```python
from build123d import *

# Parameters (mm, degrees)
SKETCH_1_W           = 32
SKETCH_1_H           = 11
EXTRUDE_1_DEPTH      = 1.6
SKETCH_2_W           = 0.64
SKETCH_2_H           = 0.64
EXTRUDE_2_DEPTH      = 6
SKETCH_3_W           = 0.64
SKETCH_3_H           = 0.64
EXTRUDE_3_DEPTH      = 8
FILLET_2_R           = 1
FILLET_3_R           = 1
FILLET_4_R           = 1
FILLET_5_R           = 1
SKETCH_4_W           = 8
SKETCH_4_H           = 11
EXTRUDE_4_DEPTH      = 8.4
FILLET_START         = 9
FILLET_4_2_OUTLINE_W = 6
FILLET_4_2_OUTLINE_H = 13
FILLET_4_2_DEPTH     = 1.960155108
FILLET_START_2       = 28.637824638
FILLET_5_2_OUTLINE_W = 5
FILLET_5_2_OUTLINE_H = 13
FILLET_5_2_DEPTH     = 2.362175362
SKETCH_5_R           = 1.25
CUT_EXTRUDE_1_DEPTH  = 6
SKETCH_6_W           = 2.5
SKETCH_6_H           = 2.5
EXTRUDE_5_DEPTH      = 2
SKETCH_7_W           = 0.64
SKETCH_7_H           = 0.64
EXTRUDE_6_DEPTH      = 5
SKETCH_8_W           = 5
SKETCH_8_H           = 6
EXTRUDE_7_DEPTH      = 1.75
SKETCH_9_W           = 1.64
SKETCH_9_H           = 1.46
EXTRUDE_8_DEPTH      = 3


with BuildPart() as part:
    # Эскиз1 → Бобышка-Вытянуть1 (new body)
    with BuildSketch(Plane(origin=(0, 0, 0), x_dir=(1, 0, 0), z_dir=(0, 1, 0))):
        with Locations((16, -5.5)):
            Rectangle(SKETCH_1_W, SKETCH_1_H)
    extrude(amount=EXTRUDE_1_DEPTH)

    # Эскиз2 → Бобышка-Вытянуть2 (add)
    with BuildSketch(Plane(origin=(0, -2, 0), x_dir=(-1, 0, 0), z_dir=(0, -1, 0))):
        with Locations((-2.32, -0.73)):
            Rectangle(SKETCH_2_W, SKETCH_2_H)
        with Locations((-2.32, -3.91)):
            Rectangle(SKETCH_2_W, SKETCH_2_H)
        with Locations((-2.32, -7.09)):
            Rectangle(SKETCH_2_W, SKETCH_2_H)
        with Locations((-2.32, -10.27)):
            Rectangle(SKETCH_2_W, SKETCH_2_H)
    extrude(amount=-EXTRUDE_2_DEPTH)

    # Эскиз3 → Бобышка-Вытянуть3 (add)
    with BuildSketch(Plane.ZY.offset(-2)):
        with Locations((0.73, 3.68)):
            Rectangle(SKETCH_3_W, SKETCH_3_H)
        with Locations((3.91, 3.68)):
            Rectangle(SKETCH_3_W, SKETCH_3_H)
        with Locations((7.09, 3.68)):
            Rectangle(SKETCH_3_W, SKETCH_3_H)
        with Locations((10.27, 3.68)):
            Rectangle(SKETCH_3_W, SKETCH_3_H)
    extrude(amount=EXTRUDE_3_DEPTH)

    # Скругление2
    fillet_2_edges = [part.edges().sort_by_distance(p)[0] for p in [
        (2.64, 4, 10.27),
    ]]
    fillet(fillet_2_edges, radius=FILLET_2_R)

    # Скругление3
    fillet_3_edges = [part.edges().sort_by_distance(p)[0] for p in [
        (2.64, 4, 0.73),
    ]]
    fillet(fillet_3_edges, radius=FILLET_3_R)

    # Fillet 4
    fillet_4_edges = [part.edges().sort_by_distance(p)[0] for p in [
        (2.64, 4, 3.91),
    ]]
    fillet(fillet_4_edges, radius=FILLET_4_R)

    # Fillet 5
    fillet_5_edges = [part.edges().sort_by_distance(p)[0] for p in [
        (2.64, 4, 7.09),
    ]]
    fillet(fillet_5_edges, radius=FILLET_5_R)

    # Эскиз4 → Бобышка-Вытянуть4 (add)
    with BuildSketch(Plane(origin=(0, 1.6, 0), x_dir=(1, 0, 0), z_dir=(0, 1, 0))):
        with Locations((28, -5.5)):
            Rectangle(SKETCH_4_W, SKETCH_4_H)
    extrude(amount=EXTRUDE_4_DEPTH)

    # Fillet 4 2: read off the stored shape, not the designer's step
    # Fillet 4 2 outline → Fillet 4 2 (cut)
    with BuildSketch(Plane(origin=(0, 0, 0), x_dir=(0.707106781186548, 0.707106781186547, 0), z_dir=(0.707106781186547, -0.707106781186548, 0)).offset(FILLET_START)):
        with Locations((24, 5.5)):
            Rectangle(FILLET_4_2_OUTLINE_W, FILLET_4_2_OUTLINE_H)
    extrude(amount=FILLET_4_2_DEPTH, mode=Mode.SUBTRACT)

    # Fillet 5 2: read off the stored shape, not the designer's step
    # Fillet 5 2 outline → Fillet 5 2 (cut)
    with BuildSketch(Plane(origin=(0, 0, 0), x_dir=(0.707106781186548, -0.707106781186547, 0), z_dir=(0.707106781186547, 0.707106781186548, 0)).offset(FILLET_START_2)):
        with Locations((15.5, -5.5)):
            Rectangle(FILLET_5_2_OUTLINE_W, FILLET_5_2_OUTLINE_H)
    extrude(amount=FILLET_5_2_DEPTH, mode=Mode.SUBTRACT)

    # Эскиз5 → Вырез-Вытянуть1 (cut)
    with BuildSketch(Plane(origin=(32, 0, 0), x_dir=(0, 0, -1), z_dir=(1, 0, 0))):
        with Locations((-8, 4.25)):
            Circle(SKETCH_5_R)
        with Locations((-3, 4.25)):
            Circle(SKETCH_5_R)
    extrude(amount=-CUT_EXTRUDE_1_DEPTH, mode=Mode.SUBTRACT)

    # Эскиз6 → Бобышка-Вытянуть5 (add)
    with BuildSketch(Plane(origin=(0, 1.6, 0), x_dir=(1, 0, 0), z_dir=(0, 1, 0))):
        with Locations((22.25, -4.21)):
            Rectangle(SKETCH_6_W, SKETCH_6_H)
        with Locations((22.25, -6.79)):
            Rectangle(SKETCH_6_W, SKETCH_6_H)
    extrude(amount=EXTRUDE_5_DEPTH)

    # Эскиз7 → Бобышка-Вытянуть6 (add)
    with BuildSketch(Plane(origin=(0, 3.6, 0), x_dir=(1, 0, 0), z_dir=(0, 1, 0))):
        with Locations((22.25, -4.21)):
            Rectangle(SKETCH_7_W, SKETCH_7_H)
        with Locations((22.25, -6.79)):
            Rectangle(SKETCH_7_W, SKETCH_7_H)
    extrude(amount=EXTRUDE_6_DEPTH)

    # Эскиз8 → Бобышка-Вытянуть7 (add)
    with BuildSketch(Plane(origin=(0, 1.6, 0), x_dir=(1, 0, 0), z_dir=(0, 1, 0))):
        with Locations((14, -5.5)):
            Rectangle(SKETCH_8_W, SKETCH_8_H)
    extrude(amount=EXTRUDE_7_DEPTH)

    # Эскиз9 → Бобышка-Вытянуть8 (add)
    with BuildSketch(Plane(origin=(0, 1.6, 0), x_dir=(1, 0, 0), z_dir=(0, 1, 0))):
        with Locations((0.82, -0.73)):
            Rectangle(SKETCH_9_W, SKETCH_9_H)
        with Locations((0.82, -3.91)):
            Rectangle(SKETCH_9_W, SKETCH_9_H)
        with Locations((0.82, -7.09)):
            Rectangle(SKETCH_9_W, SKETCH_9_H)
        with Locations((0.82, -10.27)):
            Rectangle(SKETCH_9_W, SKETCH_9_H)
    extrude(amount=EXTRUDE_8_DEPTH)


solid = part.part
```
Geometry check sheet. Reference: the model listing, model coordinates, mm. A direction names the side the tool comes from. Give positions to 0.01 mm unless a question says otherwise; leave off trailing zeros. Write each loop counter-clockwise with the first axis right and the second up, starting at its lowest first coordinate (ties: lowest second). Pieces come first, ordered by that corner, then holes.
1) Access from +Z, -Z, +X, -X, +Y, -Y to the whole of each face (thin tool, end or side, straight path). Record for faces 1 (the flat face through (14, 3.35, 5)), 2 (the flat face through (1, 3, 6.36)), 3 (the flat face through (2.3, 2.8, 6.77)), 4 (the flat face through (19.3, 0.5, 11)), 5 (the flat face through (26, 4, 8)).
2) Release check for a two-part mould opening along Z. For faces 6 (the flat face through (28, 10, 5)), 7 (the flat face through (1.64, 3, 4)), 8 (the flat face through (14, 2, 8.5)) record: pulls with the +Z half, pulls with the -Z half, needs draft (parallel to the pull), parting line crosses it, or undercut.
3) Section check B-B, the plane y = 2.5. State how many separate pieces and enclosed holes the cut face has, and give its area (3 significant figures).
4) Section check A-A, the plane x = 13. Record the boundary of the cut face in (y, z), and give its area (3 significant figures).
5) Section check C-C, the plane x = 30. Record the boundary of the cut face in (y, z), and give its area (3 significant figures).
6) Section check D-D, the plane x = 20.5. Record the boundary of the cut face in (y, z).
7) Material ranges on L1, parallel to X at y = 2, z = 4.5; L2, parallel to X at y = 2.5, z = 5; L3, parallel to Y at x = 28.1, z = 3, recorded low to high.
8) Gauge pin test, flat ends, axial feed: pin 1 (0.5 mm diameter, centred on y = -1.5, z = 0.5, fed in from -X); pin 2 (4 mm diameter, centred on x = 3.5, y = 2, fed in from +Z); pin 3 (0.7 mm diameter, centred on x = -4.5, z = 7, fed in from +Y); pin 4 (0.7 mm diameter, centred on y = -0.5, z = 4, fed in from +X). Record the tip position at first contact, or that the pin passes through.
Computed:
1. face 1: +Z, -Z, +Y
1. face 2: -X, +Y
1. face 3: +Y
1. face 4: +Z, +X, -X, +Y, -Y
1. face 5: +X
2. face 6: needs draft
2. face 7: undercut
2. face 8: pulls with the +Z half
3. separate pieces: 12
3. enclosed holes: 0
3. area: 142 mm2
4. outline: (0, 0) - (1.6, 0) - (1.6, 2.5) - (3.35, 2.5) - (3.35, 8.5) - (1.6, 8.5) - (1.6, 11) - (0, 11) - close
4. area: 28.1 mm2
5. outline: (0, 0) - (10, 0) - (10, 11) - (0, 11) - close; hole circle Ø2.5 at (4.25, 3); hole circle Ø2.5 at (4.25, 8)
5. area: 100 mm2
6. outline: (0, 0) - (1.6, 0) - (1.6, 11) - (0, 11) - close
7. L1: x = 0 to 1.64, 11.5 to 16.5, 21 to 23.5, 24 to 32
7. L2: x = 11.5 to 16.5, 21 to 23.5, 24 to 32
7. L3: y = 0 to 3, 5.5 to 10
8. pin 1: stops at x = 2
8. pin 2: stops at z = 11
8. pin 3: stops at y = 4
8. pin 4: stops at x = 2.64
